Here's how the part is built. I have some questions about the finished solid (model axes, mm). Face numbers are marked on the shaded views. A direction names the side the tool comes from. Round coordinates to 2 decimals unless told otherwise and drop trailing zeros. Order: outer loops, then holes, each group sorted by start corner. A loop starts at its lowest first (then second) coordinate and runs counter-clockwise, first axis right, second up. Notation, with made-up numbers: M 57.25,7 L 105.25,7 A33 cw 105.25,37 Z; hole C -37.5,71.25 d3. An arc over 180 degrees is marked long. Write item = value, one per line. Start each with the question number.
Item 1: Please list where these lines run through material, in increasing order: L1, parallel to X at y = 18, z = 63.5; L2, parallel to X at y = 9, z = 66.5; L3, parallel to Y at x = 32, z = 49.
Item 2: For the marked faces 1, 2, 3 and 4, which set-ups out of +Z, -Z, +X, -X, +Y, -Y let a thin tool reach every point of the face, with its end or its side?
Item 3: I want a section at A-A, the plane z = 58.5. List the corners of the cut face in (x, y) for me.
Item 4: I want a section at D-D, the plane x = 66. List the corners of the cut face in (y, z) for me, plus the area to 3 significant figures.
Item 5: I want a section at B-B, the plane y = 45.5. List the corners of the cut face in (x, z) for me, plus the area to 4 significant figures.
Item 6: I'm going to push flat-ended pins straight in: P1, Ø2.5, axis at y = 13.5, z = 16.5, coming from the -X side; P2, Ø1.5, axis at x = 38, z = 25, coming from the -Y side; P3, Ø3, axis at x = 90.5, z = 52.5, coming from the -Y side (3 decimals); P4, Ø5, axis at x = 70, y = 27.5, coming from the +Z side. Where does each tip first touch, or does it pass through?
Item 7: We'd pull the mould along X, two halves only. Please class the marked faces 5, 6, 7 and 8: pulls with the +X half, pulls with the -X half, needs draft (parallel to the pull), parting line crosses it, or undercut.
Item 8: I want a section at C-C, the plane z = 13.5. List the corners of the cut face in (x, y) for me, plus the area to 3 significant figures.
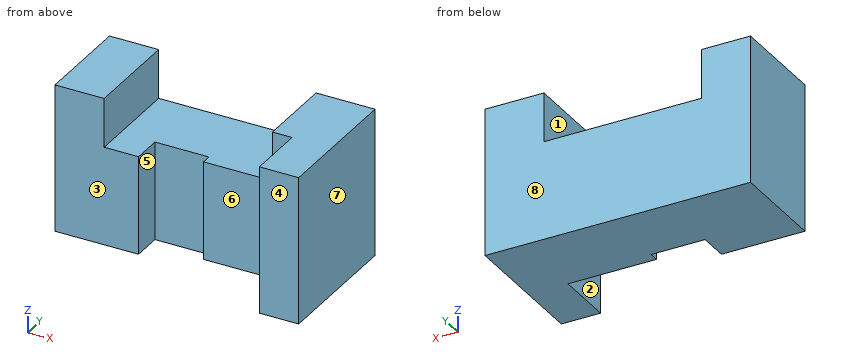
```python
from build123d import *

# Parameters (mm, degrees)
F0_W     = 25
F0_H     = 50
F1_DEPTH = 75
F3_DEPTH = 75
F5_DEPTH = 75
F6_W     = 80
F6_H     = 25
F7_DEPTH = 75
F8_W     = 10
F8_H     = 75
F9_DEPTH = 30


with BuildPart() as f1:
    # F0 (on Top) → F1 (new body)
    with BuildSketch(Plane.XY):
        with Locations((12.5, 25)):
            Rectangle(F0_W, F0_H)
    extrude(amount=F1_DEPTH)

    # F2 (on face) → F3 (join)
    with BuildSketch(Plane.XY.offset(75)):
        Polygon((25, 50), (25, 0), (42.5, 0), (42.5, 15), (70, 15), (70, 10), (105, 10), (105, 50), align=None)
    extrude(amount=-F3_DEPTH)

    # F4 (on face) → F5 (join)
    with BuildSketch(Plane.XY.offset(75)):
        Polygon((135, 50), (105, 50), (105, 10), (105, -20), (135, -20), align=None)
    extrude(amount=-F5_DEPTH)

    # F6 (on face) → F7 (cut)
    with BuildSketch(Plane.XZ.offset(20)):
        with Locations((65, 62.5)):
            Rectangle(F6_W, F6_H)
    extrude(amount=-F7_DEPTH, mode=Mode.SUBTRACT)

    # F8 (on face) → F9 (cut)
    with BuildSketch(Plane.XZ.offset(20)):
        with Locations((110, 37.5)):
            Rectangle(F8_W, F8_H)
    extrude(amount=-F9_DEPTH, mode=Mode.SUBTRACT)


solid = f1.part
```
Filled in:
q1.L1 = 0 to 25, 105 to 135
q1.L2 = 0 to 25, 115 to 135
q1.L3 = 0 to 50
q2.face_1 = +Z, +Y, -Y
q2.face_2 = +Z, -Z, -Y
q2.face_3 = +Z, -Z, -X, -Y
q2.face_4 = +Z, -Z, +X, -X, -Y
q3.outline = M 0,0 L 25,0 L 25,50 L 0,50 Z; M 105,10 L 115,10 L 115,-20 L 135,-20 L 135,50 L 105,50 Z
q4.outline = M 15,0 L 50,0 L 50,50 L 15,50 Z
q4.area = 1,750 mm^2
q5.outline = M 0,0 L 135,0 L 135,75 L 105,75 L 105,50 L 25,50 L 25,75 L 0,75 Z
q5.area = 8,125 mm^2
q6.P1 = 0
q6.P2 = 0
q6.P3 = through
q6.P4 = 50
q7.face_5 = undercut
q7.face_6 = undercut
q7.face_7 = pulls with the +X half
q7.face_8 = needs draft
q8.outline = M 0,0 L 42.5,0 L 42.5,15 L 70,15 L 70,10 L 115,10 L 115,-20 L 135,-20 L 135,50 L 0,50 Z
q8.area = 6,290 mm^2
